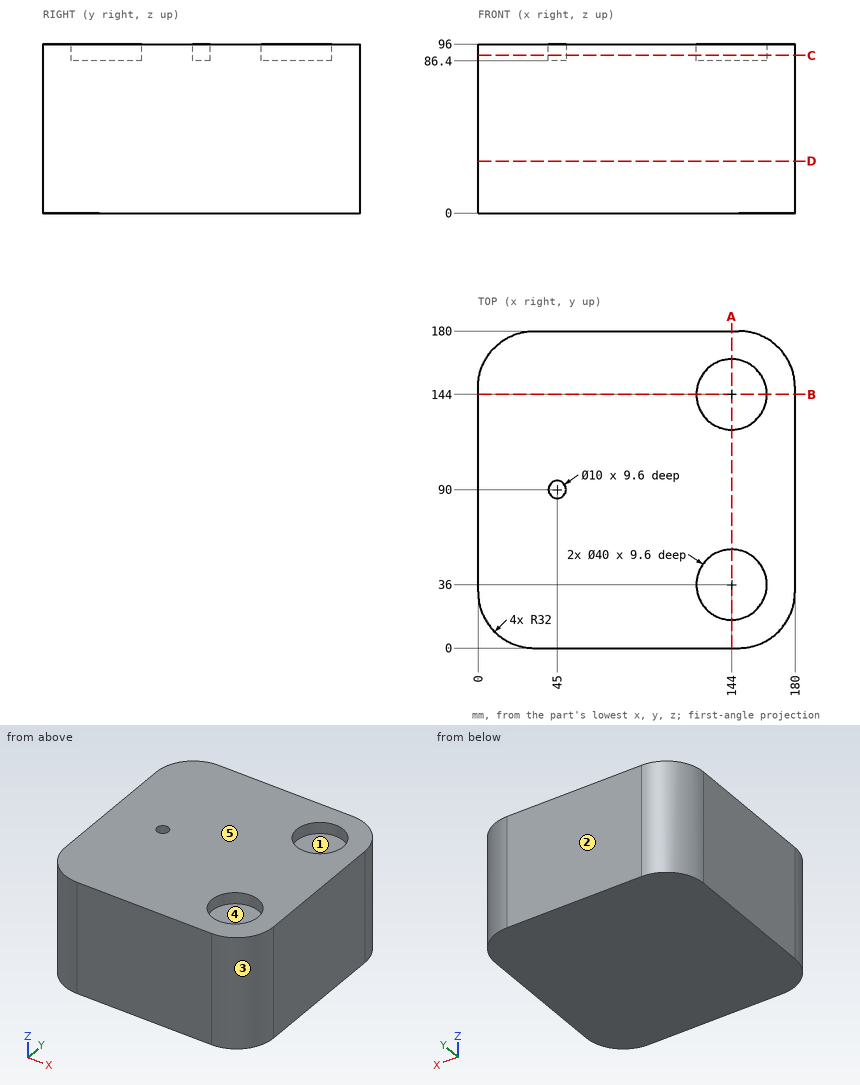
Answer from the drawing. Dimensions are ordinates in mm from the lowest x, y and z of the part. A direction names the side the tool comes from. Round coordinates to 2 decimals unless told otherwise and drop trailing zeros. Order: outer loops, then holes, each group sorted by start corner. A loop starts at its lowest first (then second) coordinate and runs counter-clockwise, first axis right, second up. Notation, with made-up numbers: (26, 47) - (80, 47) arc R23 ccw to (80, 67) - close; hole circle Ø9 at (88, 32). An arc over 180 degrees is marked (long way). Put each result on its own line as item: value. Start each with the question number.
(1) Straight lines are drawn through the part: probe 1 along Y at (x, z) = (144, 90); probe 2 along Y at (x, z) = (45, 92.75); probe 3 along Y at (x, z) = (161, 86.5). For each, find the intervals that lie inside material, in ascending order. Write a range as from..to.
(2) Find section A-A (x = 144). Give the vertices of the cut face in (y, z), plus the area to 3 significant figures.
(3) For the marked faces 4 and 5, determine the directions among +Z, -Z, +X, -X, +Y, -Y from which every point of the face is accessible in a straight line to the end or side of a thin tool.
(4) Find section D-D (z = 29.5). Give the vertices of the cut face in (x, y), plus the area to 3 significant figures.
(5) Find section C-C (z = 89.5). Give the vertices of the cut face in (x, y), plus the area to 3 significant figures.
(6) Determine the mould class of the marked faces 1, 2 and 3 for opening direction Y: released by +Y, released by -Y, zero draft, split by the parting line, or undercut.
(7) Given P1, Ø12, axis at x = 140.5, y = 141, coming from the +Z side; P2, Ø2, axis at y = 23.5, z = 60.5, coming from the -X side, each flat-ended and moving along its own axis, determine where each tip first touches the part or whether it passes through.
(8) Find section B-B (y = 144). Give the vertices of the cut face in (x, z).
Reply:
1. probe 1: 0..16, 56..124, 164..180
1. probe 2: 0..85, 95..180
1. probe 3: 2.76..25.46, 46.54..133.46, 154.54..177.24
2. outline: (0, 0) - (180, 0) - (180, 96) - (164, 96) - (164, 86.4) - (124, 86.4) - (124, 96) - (56, 96) - (56, 86.4) - (16, 86.4) - (16, 96) - (0, 96) - close
2. area: 16,500 mm^2
3. face 4: +Z
3. face 5: +Z, +X, -X, +Y, -Y
4. outline: (0, 32) arc R32 ccw to (32, 0) - (148, 0) arc R32 ccw to (180, 32) - (180, 148) arc R32 ccw to (148, 180) - (32, 180) arc R32 ccw to (0, 148) - close
4. area: 31,500 mm^2
5. outline: (0, 32) arc R32 ccw to (32, 0) - (148, 0) arc R32 ccw to (180, 32) - (180, 148) arc R32 ccw to (148, 180) - (32, 180) arc R32 ccw to (0, 148) - close; hole circle Ø10 at (45, 90); hole circle Ø40 at (144, 36); hole circle Ø40 at (144, 144)
5. area: 28,900 mm^2
6. face 1: undercut
6. face 2: released by +Y
6. face 3: released by -Y
7. P1: z = 86.4
7. P2: x = 0.89
8. outline: (0, 0) - (180, 0) - (180, 96) - (164, 96) - (164, 86.4) - (124, 86.4) - (124, 96) - (0, 96) - close
